from build123d import *

# Parameters (mm, degrees)
BOSS_EXTRUDE1_DEPTH = 3
SKETCH2_W           = 3
SKETCH2_H           = 3
SKETCH2_H_2         = 36.5
SKETCH2_W_2         = 36.5
SKETCH2_W_3         = 29
SKETCH2_H_3         = 29
CUT_EXTRUDE2_DEPTH  = 3
SKETCH3_R           = 1.47
CUT_EXTRUDE3_DEPTH  = 3
SKETCH4_W           = 16
SKETCH4_H           = 3
CUT_EXTRUDE6_DEPTH  = 3
SKETCH6_W           = 16
SKETCH6_H           = 3
CUT_EXTRUDE7_DEPTH  = 3
SKETCH7_W           = 3
SKETCH7_H           = 3
CUT_EXTRUDE8_DEPTH  = 3


with BuildPart() as part:
    # Sketch1 → Boss-Extrude1 (new body)
    with BuildSketch(Plane(origin=(0, 0, 0), x_dir=(1, 0, 0), z_dir=(0, 1, 0))):
        Polygon((70, 70), (-70, 70), (0, 0), align=None)
        Polygon((0, 0), (-70, 70), (-70, -70), align=None)
        Polygon((70, -70), (0, 0), (-70, -70), align=None)
        Polygon((70, 70), (0, 0), (70, -70), align=None)
    extrude(amount=BOSS_EXTRUDE1_DEPTH)

    # Sketch2 → Cut-Extrude2 (cut)
    with BuildSketch(Plane(origin=(0, 3, 0), x_dir=(1, 0, 0), z_dir=(0, 1, 0))):
        with Locations((-68.5, 68.5)):
            Rectangle(SKETCH2_W, SKETCH2_H)
        with Locations((-68.5, 48.75)):
            Rectangle(SKETCH2_W, SKETCH2_H_2)
        with Locations((-48.75, 68.5)):
            Rectangle(SKETCH2_W_2, SKETCH2_H)
        with Locations((48.75, 68.5)):
            Rectangle(SKETCH2_W_2, SKETCH2_H)
        with Locations((68.5, 68.5)):
            Rectangle(SKETCH2_W, SKETCH2_H)
        with Locations((68.5, 48.75)):
            Rectangle(SKETCH2_W, SKETCH2_H_2)
        with Locations((68.5, -68.5)):
            Rectangle(SKETCH2_W, SKETCH2_H)
        with Locations((68.5, -48.75)):
            Rectangle(SKETCH2_W, SKETCH2_H_2)
        with Locations((48.75, -68.5)):
            Rectangle(SKETCH2_W_2, SKETCH2_H)
        with Locations((-48.75, -68.5)):
            Rectangle(SKETCH2_W_2, SKETCH2_H)
        with Locations((-68.5, -68.5)):
            Rectangle(SKETCH2_W, SKETCH2_H)
        with Locations((-68.5, -48.75)):
            Rectangle(SKETCH2_W, SKETCH2_H_2)
        with Locations((0, 68.5)):
            Rectangle(SKETCH2_W_3, SKETCH2_H)
        with Locations((0, -68.5)):
            Rectangle(SKETCH2_W_3, SKETCH2_H)
        with Locations((68.5, 0)):
            Rectangle(SKETCH2_W, SKETCH2_H_3)
        with Locations((-68.5, 0)):
            Rectangle(SKETCH2_W, SKETCH2_H_3)
    extrude(amount=-CUT_EXTRUDE2_DEPTH, mode=Mode.SUBTRACT)

    # Sketch3 → Cut-Extrude3 (cut)
    with BuildSketch(Plane(origin=(0, 3, 0), x_dir=(1, 0, 0), z_dir=(0, 1, 0))):
        with Locations((22.5, -68.5)):
            Circle(SKETCH3_R)
        with Locations((-22.5, -68.5)):
            Circle(SKETCH3_R)
        with Locations((-22.5, 68.5)):
            Circle(SKETCH3_R)
        with Locations((22.5, 68.5)):
            Circle(SKETCH3_R)
        with Locations((68.5, -22.5)):
            Circle(SKETCH3_R)
        with Locations((-68.5, -22.5)):
            Circle(SKETCH3_R)
        with Locations((-68.5, 22.5)):
            Circle(SKETCH3_R)
        with Locations((68.5, 22.5)):
            Circle(SKETCH3_R)
    extrude(amount=-CUT_EXTRUDE3_DEPTH, mode=Mode.SUBTRACT)

    # Sketch4 → Cut-Extrude6 (cut)
    with BuildSketch(Plane(origin=(0, 3, 0), x_dir=(1, 0, 0), z_dir=(0, 1, 0))):
        with Locations((22.5, 68.5)):
            Rectangle(SKETCH4_W, SKETCH4_H)
    extrude(amount=-CUT_EXTRUDE6_DEPTH, mode=Mode.SUBTRACT)

    # Sketch6 → Cut-Extrude7 (cut)
    with BuildSketch(Plane(origin=(0, 3, 0), x_dir=(1, 0, 0), z_dir=(0, 1, 0))):
        with Locations((-22.5, 68.5)):
            Rectangle(SKETCH6_W, SKETCH6_H)
    extrude(amount=-CUT_EXTRUDE7_DEPTH, mode=Mode.SUBTRACT)

    # Sketch7 → Cut-Extrude8 (cut)
    with BuildSketch(Plane(origin=(0, 3, 0), x_dir=(1, 0, 0), z_dir=(0, 1, 0))):
        with Locations((35.5, 33.5)):
            Rectangle(SKETCH7_W, SKETCH7_H)
        with Locations((35.5, 60.5)):
            Rectangle(SKETCH7_W, SKETCH7_H)
    extrude(amount=-CUT_EXTRUDE8_DEPTH, mode=Mode.SUBTRACT)


solid = part.part
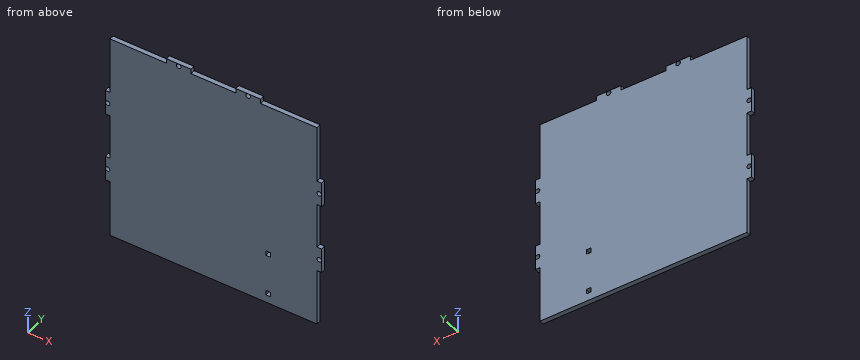
The model under review builds one solid part; all positions refer to its coordinate system, in mm. Round coordinates to 2 decimals unless told otherwise and drop trailing zeros. Order: outer loops, then holes, each group sorted by start corner. A loop starts at its lowest first (then second) coordinate and runs counter-clockwise, first axis right, second up. Notation, with made-up numbers: (44.5, 77) -> (53.5, 77) arc R7 ccw to (53.5, 81) -> close; hole circle Ø8 at (58, 88.5). An arc over 180 degrees is marked (long way). Return JSON: item names as keys, results as strings.
1. Take a section at B-B (z = 0.5). Write out the cut boundary in (x, y).
Answer block:
{"outline": "(-67, 0) -> (67, 0) -> (67, 3) -> (-67, 3) -> close"}
2. Take a section at A-A (y = 2.1). State how many separate pieces and enclosed holes the cut face has, then the cut area to 3 significant figures.
Answer block:
{"separate pieces": "1", "enclosed holes": "8", "area": "18,200 mm²"}
3. For L1, parallel to X at y = 2.3, z = 68.5; L2, parallel to Z at x = 63, y = 0.2, list the stretches that pass through material, from the lowest coordinate up. Write a range as [from, to].
Answer block:
{"L1": "x = [-30.5, -23.97], [-21.03, -14.5], [14.5, 21.03], [23.97, 30.5]", "L2": "z = [-67, 67]"}
4. Insertion check: P1, Ø1.5, axis at x = -42, z = 32.5, coming from the -Y side; P2, Ø1.5, axis at y = 2, z = 44, coming from the +X side; P3, Ø0.9, axis at y = 1.5, z = -34, coming from the -X side. Each pin has a flat end and moves straight along its axis. Give the tip position at first contact, or say it passes through.
Answer block:
{"P1": "stops at y = 0", "P2": "stops at x = 67", "P3": "stops at x = -67"}
5. Take a section at C-C (x = 46.5). Write out the cut boundary in (y, z), then the cut area to 3 significant figures.
Answer block:
{"outline": "(0, -67) -> (3, -67) -> (3, 67) -> (0, 67) -> close", "area": "402 mm²"}
